from build123d import *

# Parameters (mm, degrees)
SKETCH1_W           = 12
SKETCH1_H           = 12
BOSS_EXTRUDE1_DEPTH = 3.5
SKETCH2_R           = 2.5
BOSS_EXTRUDE2_DEPTH = 1
SKETCH3_R           = 0.5
BOSS_EXTRUDE3_DEPTH = 0.5
SKETCH4_W           = 2
SKETCH4_H           = 2
BOSS_EXTRUDE4_DEPTH = 1
SKETCH5_W           = 3.8
SKETCH5_H           = 3.8
BOSS_EXTRUDE5_DEPTH = 1
SKETCH6_R           = 0.75
BOSS_EXTRUDE6_DEPTH = 3.5


with BuildPart() as part:
    # Sketch1 → Boss-Extrude1 (new body)
    with BuildSketch(Plane(origin=(0, 0, 0), x_dir=(1, 0, 0), z_dir=(0, 1, 0))):
        Rectangle(SKETCH1_W, SKETCH1_H)
    extrude(amount=BOSS_EXTRUDE1_DEPTH)

    # Sketch2 → Boss-Extrude2 (add)
    with BuildSketch(Plane(origin=(0, 3.5, 0), x_dir=(1, 0, 0), z_dir=(0, 1, 0))):
        Circle(SKETCH2_R)
    extrude(amount=BOSS_EXTRUDE2_DEPTH)

    # Sketch3 → Boss-Extrude3 (add)
    with BuildSketch(Plane(origin=(0, 3.5, 0), x_dir=(1, 0, 0), z_dir=(0, 1, 0))):
        with Locations((-4.51726096, 4.56041336)):
            Circle(SKETCH3_R)
        with Locations((-4.51726096, -4.43958664)):
            Circle(SKETCH3_R)
        with Locations((4.48273904, -4.43958664)):
            Circle(SKETCH3_R)
        with Locations((4.48273904, 4.56041336)):
            Circle(SKETCH3_R)
    extrude(amount=BOSS_EXTRUDE3_DEPTH)

    # Sketch4 → Boss-Extrude4 (add)
    with BuildSketch(Plane(origin=(0, 4.5, 0), x_dir=(1, 0, 0), z_dir=(0, 1, 0))):
        Rectangle(SKETCH4_W, SKETCH4_H)
    extrude(amount=BOSS_EXTRUDE4_DEPTH)

    # Sketch5 → Boss-Extrude5 (add)
    with BuildSketch(Plane(origin=(0, 5.5, 0), x_dir=(1, 0, 0), z_dir=(0, 1, 0))):
        Rectangle(SKETCH5_W, SKETCH5_H)
    extrude(amount=BOSS_EXTRUDE5_DEPTH)

    # Sketch6 → Boss-Extrude6 (add)
    with BuildSketch(Plane.XZ):
        with Locations((-5.25, 2.5)):
            Circle(SKETCH6_R)
        with Locations((-5.25, -2.5)):
            Circle(SKETCH6_R)
        with Locations((5.25, -2.5)):
            Circle(SKETCH6_R)
        with Locations((5.25, 2.5)):
            Circle(SKETCH6_R)
    extrude(amount=BOSS_EXTRUDE6_DEPTH)


solid = part.part
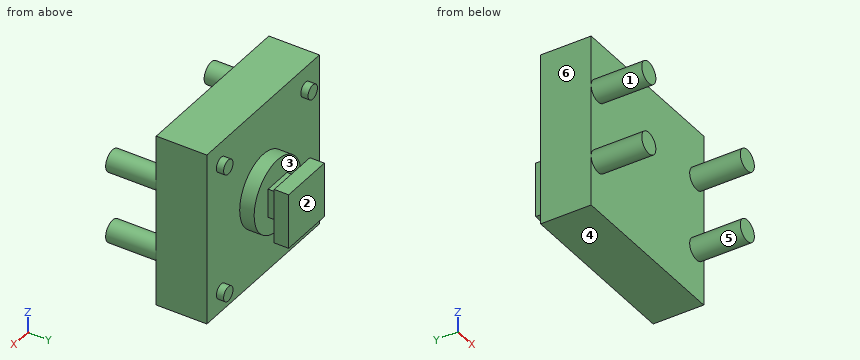
For this review, take the finished solid that the model builds, in its own axes (mm). Face numbers are marked on the shaded views. A direction names the side the tool comes from. Round coordinates to 2 decimals unless told otherwise and drop trailing zeros. Loops run counter-clockwise (first coordinate to the right, second up) from the corner with the lowest first, then second, coordinate; pieces in that order, holes last. Notation, with made-up numbers: (-23, -10.5) - (-18, -10.5) arc R20 cw to (-18, 11.5) - close; hole circle Ø7 at (86, 48.5). An arc over 180 degrees is marked (long way). Use one line per item in the form item = value.
Item 1: Consider section C-C on x = 5.25. Write out the cut boundary in (y, z).
Answers:
outline = (-3.5, -3.25) - (0, -3.25) - (0, -6) - (3.5, -6) - (3.5, 6) - (0, 6) - (0, 3.25) - (-3.5, 3.25) - (-3.5, 1.75) - (0, 1.75) - (0, -1.75) - (-3.5, -1.75) - close
Item 2: Consider section B-B on z = 0. Write out the cut boundary in (x, y).
Answers:
outline = (-6, 0) - (6, 0) - (6, 3.5) - (2.5, 3.5) - (2.5, 4.5) - (1, 4.5) - (1, 5.5) - (1.9, 5.5) - (1.9, 6.5) - (-1.9, 6.5) - (-1.9, 5.5) - (-1, 5.5) - (-1, 4.5) - (-2.5, 4.5) - (-2.5, 3.5) - (-6, 3.5) - close
Item 3: Clearance check with flat-ended pins moving along their axes: P1, Ø1, axis at x = 2, z = -3.5, coming from the +Y side; P2, Ø1.1, axis at y = 5, z = 0, coming from the +X side; P3, Ø0.5, axis at y = 5, z = 0, coming from the -X side. State where each tip first meets the part, or that it passes through.
Answers:
P1 = 3.5
P2 = 2.5
P3 = -1
Item 4: Mouldability with a two-part tool opening along X and no side actions: class the marked faces 4, 5 and 6 as +X half, -X half, draft (parallel to the pull), parting line (faces both ways), or undercut.
Answers:
face_4 = draft
face_5 = undercut
face_6 = -X half
Item 5: Tool access review of the marked faces 1, 2 and 3: name each direction out of +Z, -Z, +X, -X, +Y, -Y from which nothing blocks a thin tool from reaching the whole face with its end or side.
Answers:
face_1 = -Y
face_2 = +Z, -Z, +X, -X, +Y
face_3 = none
Item 6: For line 1 (Z direction, x = -5.25, y = -1.25); line 2 (X direction, y = 3.75, z = -4.5); line 3 (Y direction, x = 4, z = 5.5), list the stretches that pass through material, from the lowest coordinate up.
Answers:
line_1 = -3.25 to -1.75, 1.75 to 3.25
line_2 = -5.01 to -4.02, 3.99 to 4.98
line_3 = 0 to 3.5
Item 7: Consider section D-D on y = 5. Write out the cut boundary in (x, z).
Answers:
outline = (-1, -1) - (1, -1) - (1, 1) - (-1, 1) - close
Item 8: Consider section A-A on x = 0. Write out the cut boundary in (y, z), then the cut area to 3 significant figures.
Answers:
outline = (0, -6) - (3.5, -6) - (3.5, -2.5) - (4.5, -2.5) - (4.5, -1) - (5.5, -1) - (5.5, -1.9) - (6.5, -1.9) - (6.5, 1.9) - (5.5, 1.9) - (5.5, 1) - (4.5, 1) - (4.5, 2.5) - (3.5, 2.5) - (3.5, 6) - (0, 6) - close
area = 52.8 mm^2
